The model under review builds one solid part; all positions refer to its coordinate system, in mm. A direction names the side the tool comes from. Coordinates: 2 decimals unless noted, no trailing zeros. Write each loop counter-clockwise with the first axis right and the second up, starting at its lowest first coordinate (ties: lowest second). Pieces come first, ordered by that corner, then holes. Notation, with made-up numbers: (40.25, 23) - (44.25, 23) arc R9 cw to (44.25, 30) - close; hole circle Ø10 at (69, -4). An arc over 180 degrees is marked (long way). Put each result on its own line as item: value. Start each with the question number.
Item 1: Mouldability with a two-part tool opening along Y and no side actions: class faces 4 (the face through (135.094, 360.616, 292.05)), 5 (the face through (207, 286, 292)), 6 (the face through (166.983, 336.468, 292.05)) as pulls with the +Y half, pulls with the -Y half, needs draft (parallel to the pull), parting line crosses it, or undercut.
Item 2: Consider section C-C on y = 474.5. Give the boundary of the cut face in (x, z).
Item 3: Consider section A-A on z = 232.5. Give the boundary of the cut face in (x, y), then the cut area to 3 significant figures.
Item 4: Consider section B-B on x = 203. Give the boundary of the cut face in (y, z).
Item 5: For pin 1 (4 mm diameter, centred on x = 144, z = 302, fed in from +Y); pin 2 (6 mm diameter, centred on y = 474, z = 306.5, fed in from -X); pin 3 (4 mm diameter, centred on y = 347.5, z = 309.5, fed in from -X), all flat-tipped, find the tip position at first contact; note any pin that passes through.
Item 6: To check wall thickness, follow L1, parallel to Y at x = 101, z = 223.5; L2, parallel to Y at x = 63, z = 286; L3, parallel to X at y = 423, z = 297.5. State the ranges of each line that lie inside material, in increasing order. Write a range as [from, to].
Item 7: Machinability: for faces 1 (the face through (-26.846, 472.414, 292.05)), 2 (the face through (38.924, 432.389, 292.05)), 3 (the face through (67, 391, 216)), which of the approach directions +Z, -Z, +X, -X, +Y, -Y give a long, thin tool a straight path to every point of the face, cutting with its end or side? Answer none if there is none.
```python
from build123d import *

# Parameters (mm, degrees)
EXTRUDE_1_DEPTH = 150


with BuildPart() as part:
    # 草图1 → 凸台-拉伸1 (new body)
    with BuildSketch(Plane.XY.offset(366)):
        Polygon((-87.024672103, 495), (192, 286), (222.024672103, 286), (-57, 495), align=None)
        Polygon((2.475382036, 450.450696342), (34.490163642, 426.470417805), (43.482768093, 438.475960908), (11.467986487, 462.456239445), align=None)
        Polygon((130.534508461, 354.529582195), (162.549290067, 330.549303658), (171.541894518, 342.55484676), (139.527112912, 366.535125297), align=None)
    extrude(amount=-EXTRUDE_1_DEPTH)


solid = part.part
```
Report:
1. face 4: pulls with the +Y half
1. face 5: pulls with the -Y half
1. face 6: undercut
2. outline: (-59.66, 216) - (-29.63, 216) - (-29.63, 366) - (-59.66, 366) - close
3. outline: (-87.02, 495) - (192, 286) - (222.02, 286) - (162.55, 330.55) - (171.54, 342.55) - (139.53, 366.54) - (130.53, 354.53) - (34.49, 426.47) - (43.48, 438.48) - (11.47, 462.46) - (2.48, 450.45) - (-57, 495) - close
3. area: 7,480 mm²
4. outline: (286, 216) - (300.25, 216) - (300.25, 366) - (286, 366) - close
5. pin 1: y = 364.68
5. pin 2: x = -62.99
5. pin 3: x = 107.22
6. L1: [354.16, 376.65]
6. L2: [382.63, 405.12]
6. L3: [9.1, 39.12]
7. face 1: +Z, -Z, +Y
7. face 2: +Z, -Z, +X
7. face 3: -Z, +X, -X, +Y, -Y
